Check sheet for the modelled part. Datum: model origin and axes. Units: mm. Face numbers are marked on the shaded views. Round coordinates to 2 decimals unless told otherwise and drop trailing zeros. Order: outer loops, then holes, each group sorted by start corner. A loop starts at its lowest first (then second) coordinate and runs counter-clockwise, first axis right, second up. Notation, with made-up numbers: M 23,19 L 82,19 A26 cw 82,46 Z; hole C -32,2.25 d2. An arc over 180 degrees is marked long. One line per item, written item: value. Start each with the question number.
(1) Cross-section at A-A, the plane z = 0. Enter the section's corners in (x, y).
(2) Release check for a two-part mould opening along Z. For the marked faces 1 and 2 record: released by +Z, released by -Z, zero draft, split by the parting line, or undercut.
(3) Cross-section at B-B, the plane y = 0. Enter the section's corners in (x, z).
(4) Thickness scan on L1, parallel to Y at x = 100, z = 0; L2, parallel to Z at x = 105, y = 6. Record the ranges inside material, lowest first.
(5) Depth check by flat-ended pin: pin 1 Ø1.5 at (x, y) = (58, -1) entering from +Z; pin 2 Ø1.5 at (x, z) = (136.5, -6.5) entering from -Y; pin 3 Ø12 at (x, y) = (92, 8) entering from -Z; pin 4 Ø2 at (y, z) = (-8, -5.5) entering from -X. Enter the tip coordinate at first touch or a pass-through.
(6) Cross-section at D-D, the plane x = 91. Enter the section's corners in (y, z).
(7) Cross-section at C-C, the plane y = 7. Enter the section's corners in (x, z), and give its area (3 significant figures).
from build123d import *

# Parameters (mm, degrees)
CROQUIS1_R              = 10.5
SALIENTE_EXTRUIR1_DEPTH = 155
CROQUIS2_R              = 10
CORTAR_EXTRUIR1_DEPTH   = 155
CROQUIS3_R              = 3.25
CORTAR_EXTRUIR2_DEPTH   = 2.5


with BuildPart() as part:
    # Croquis1 → Saliente-Extruir1 (new body)
    with BuildSketch(Plane(origin=(0, 0, 0), x_dir=(0, 0, -1), z_dir=(1, 0, 0))):
        Circle(CROQUIS1_R)
    extrude(amount=SALIENTE_EXTRUIR1_DEPTH)

    # Croquis2 → Cortar-Extruir1 (cut)
    with BuildSketch(Plane(origin=(155, 0, 0), x_dir=(0, 0, -1), z_dir=(1, 0, 0))):
        Circle(CROQUIS2_R)
    extrude(amount=-CORTAR_EXTRUIR1_DEPTH, mode=Mode.SUBTRACT)

    # Croquis3 → Cortar-Extruir2 (cut, symmetric)
    with BuildSketch(Plane.XY.offset(10.369970807)):
        with Locations((130, 0)):
            Circle(CROQUIS3_R)
    extrude(amount=CORTAR_EXTRUIR2_DEPTH, both=True, mode=Mode.SUBTRACT)


solid = part.part
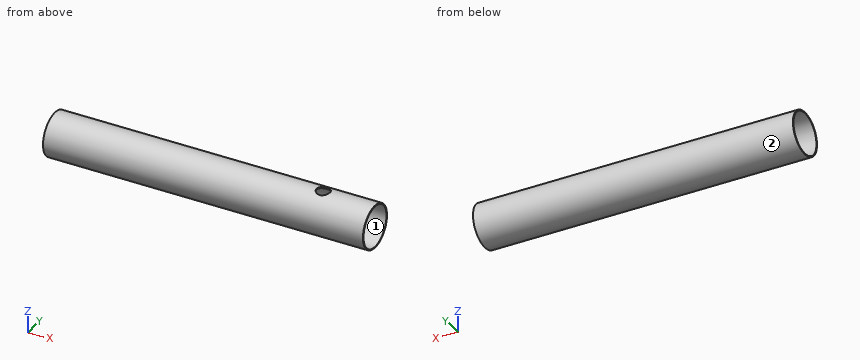
Values found:
1. outline: M 0,-10.5 L 155,-10.5 L 155,-10 L 0,-10 Z; M 0,10 L 155,10 L 155,10.5 L 0,10.5 Z
2. face 1: undercut
2. face 2: split by the parting line
3. outline: M 0,-10.5 L 155,-10.5 L 155,-10 L 0,-10 Z; M 0,10 L 126.75,10 L 126.75,10.5 L 0,10.5 Z; M 133.25,10 L 155,10 L 155,10.5 L 133.25,10.5 Z
4. L1: -10.5 to -10, 10 to 10.5
4. L2: -8.62 to -8, 8 to 8.62
5. pin 1: z = 10.5
5. pin 2: y = -8.79
5. pin 3: z = -10.31
5. pin 4: x = 0
6. outline: C 0,0 d21; hole C 0,0 d20
7. outline: M 0,-7.83 L 155,-7.83 L 155,-7.14 L 0,-7.14 Z; M 0,7.14 L 155,7.14 L 155,7.83 L 0,7.83 Z
7. area: 212 mm^2
